Source: CAD feature listing. Evaluate the final solid. Frame: model axes, mm. A direction names the side the tool comes from. Round coordinates to 2 decimals unless told otherwise and drop trailing zeros. Write each loop counter-clockwise with the first axis right and the second up, starting at its lowest first coordinate (ties: lowest second). Pieces come first, ordered by that corner, then holes. Notation, with made-up numbers: M 3.5,34.25 L 17.5,34.25 A31 ccw 17.5,73.25 Z; hole C 47,20 d1. An arc over 180 degrees is marked long. Answer in a Markdown table with one row per item.
from build123d import *

# Parameters (mm, degrees)
F1_DEPTH = 20


with BuildPart() as f1:
    # F0 (on Front) → F1 (new body)
    with BuildSketch(Plane.XZ):
        Polygon((-46, -5), (-41.750403, 0), (-46, 0), align=None)
        Polygon((0, -5), (0, 0), (-41.750403, 0), (-46, -5), align=None)
        Polygon((-46, 0), (-41.750403, 0), (-29.162069, 14.811211), (-29.162069, 19.811211), align=None)
        Polygon((16.837931, 19.811211), (0, 0), (0, -5), (16.837931, 14.811211), align=None)
    extrude(amount=F1_DEPTH)


solid = f1.part
Q1. Section C-C (x = -7.5). Return loops of the section in (y, z).
Solutions:
| item | result |
|---|---|
| outline | M -20,-5 L 0,-5 L 0,0 L -20,0 Z |
Q2. Section A-A (y = -10.25). Return loops of the section in (x, z).
Solutions:
| item | result |
|---|---|
| outline | M -46,-5 L 0,-5 L 16.84,14.81 L 16.84,19.81 L 0,0 L -41.75,0 L -29.16,14.81 L -29.16,19.81 L -46,0 Z |
Q3. Material intervals for probe 1 along X at (y, z) = (-18, 16.75); probe 2 along X at (y, z) = (-13.75, 18.75); probe 3 along Z at (x, y) = (-24, -1.25), sorted ascending.
Solutions:
| item | result |
|---|---|
| probe 1 | x = -31.76 to -29.16, 14.24 to 16.84 |
| probe 2 | x = -30.06 to -29.16, 15.94 to 16.84 |
| probe 3 | z = -5 to 0 |
Q4. Section D-D (z = 15.5). Return loops of the section in (x, y).
Solutions:
| item | result |
|---|---|
| outline | M -32.83,-20 L -29.16,-20 L -29.16,0 L -32.83,0 Z; M 13.17,-20 L 16.84,-20 L 16.84,0 L 13.17,0 Z |
Q5. Section B-B (z = 6.75). Return loops of the section in (x, y).
Solutions:
| item | result |
|---|---|
| outline | M -40.26,-20 L -36.01,-20 L -36.01,0 L -40.26,0 Z; M 5.74,-20 L 9.99,-20 L 9.99,0 L 5.74,0 Z |
Q6. Contact query for flat-ended pins moving along their axis: pin 1 Ø10 at (x, y) = (-25.5, -7.5) entering from +Z; pin 2 Ø10 at (y, z) = (-11.5, 9.5) entering from +X; pin 3 Ø1.5 at (x, z) = (-32.5, 8.5) entering from -Y; pin 4 Ø1.5 at (x, y) = (-19, -15) entering from +Z. Output: stop coordinate, or through.
Solutions:
| item | result |
|---|---|
| pin 1 | stops at z = 19.81 |
| pin 2 | stops at x = 16.57 |
| pin 3 | passes through |
| pin 4 | stops at z = 0 |
Q7. Access query for faces 1 (the flat face through (-19, -20, -1)), 2 (the flat face through (-35.544, -9.86, 7.302)), 3 (the flat face through (8.5, -9.9, 10)). Directions: +Z, -Z, +X, -X, +Y, -Y. A direction counts if a zero-diameter tool reaches every point of the face in a straight line with its end or side. Return the directions, or none.
Solutions:
| item | result |
|---|---|
| face 1 | +Z, -Z, +X, -X, -Y |
| face 2 | +Y, -Y |
| face 3 | +Z, +Y, -Y |
